Verification items for the finished model (mm, model axes). Face numbers are marked on the shaded views. A direction names the side the tool comes from. Give positions to 0.01 mm unless a question says otherwise; leave off trailing zeros. Order: outer loops, then holes, each group sorted by start corner. A loop starts at its lowest first (then second) coordinate and runs counter-clockwise, first axis right, second up. Notation, with made-up numbers: (20, 68.25) -> (78, 68.25) arc R9 ccw to (78, 78.25) -> close; hole circle Ø2 at (76, 17). An arc over 180 degrees is marked (long way). Return JSON: item names as keys, results as strings. Group by question number.
(1) Cross-section at C-C on y = 15. Enter the section's corners in (x, z), then the cut area to 3 significant figures.
(2) Cross-section at B-B on x = 1. Enter the section's corners in (y, z).
(3) Depth check by flat-ended pin: pin 1 Ø2.5 at (x, y) = (11, 19.05) entering from -Z; pin 2 Ø3 at (x, y) = (12.5, 19.5) entering from -Z; pin 3 Ø12 at (x, z) = (8.5, 5) entering from +Y; pin 4 Ø8 at (x, z) = (1, 24.5) entering from -Y. Enter the tip coordinate at first touch or a pass-through.
(4) Tool access check on the marked faces 1 and 2. Record the directions out of +Z, -Z, +X, -X, +Y, -Y that give a thin tool (end or side, any length) a straight path to the whole face; none if there is none.
(5) Cross-section at A-A on y = 0. Enter the section's corners in (x, z), then the cut area to 3 significant figures.
(6) Cross-section at D-D on x = -3.5. Enter the section's corners in (y, z), then the cut area to 3 significant figures.
(7) Thickness scan on line 1 along Y through (x, z) = (-11, 36); line 2 along Z through (x, y) = (0, -17.5); line 3 along X through (y, z) = (-10.5, 35). Record the ranges inside material, lowest first.
(8) Release check for a two-part mould opening along Y. For the marked faces 3, 4 and 5 record: pulls with the +Y half, pulls with the -Y half, needs draft (parallel to the pull), parting line crosses it, or undercut.
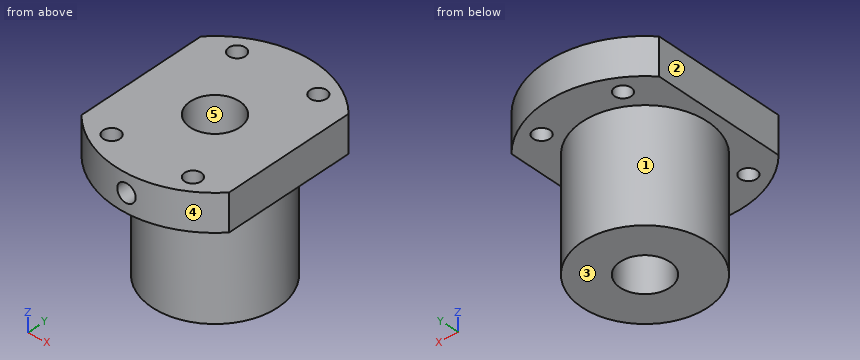
from build123d import *

# Parameters (mm, degrees)
SKETCH1_R                        = 17
BOSS_EXTRUDE1_DEPTH              = 30
BOSS_EXTRUDE2_DEPTH              = 10
SKETCH4_R                        = 6.71
CUT_EXTRUDE1_DEPTH               = 53.239831546
TAP_DRILL_FOR_M6X1_0_TAP1_REACH  = 72.114
TAP_DRILL_FOR_M6X1_0_TAP1_BORE_R = 2.5
F_4_5_4_5_DIAMETER_HOLE1_D       = 4.5


with BuildPart() as part:
    # Sketch1 → Boss-Extrude1 (new body)
    with BuildSketch(Plane.XY):
        Circle(SKETCH1_R)
    extrude(amount=BOSS_EXTRUDE1_DEPTH)

    # Sketch3 → Boss-Extrude2 (add)
    with BuildSketch(Plane.XY.offset(30)):
        with BuildLine():
            Line((-20, -18.138357147), (-20, 18.138357147))
            ThreePointArc((-20, 18.138357147), (0, 27), (20, 18.138357147))
            Line((20, 18.138357147), (20, -18.138357147))
            ThreePointArc((20, -18.138357147), (0, -27), (-20, -18.138357147))
        make_face()
    extrude(amount=BOSS_EXTRUDE2_DEPTH)

    # Sketch4 → Cut-Extrude1 (cut, through all)
    with BuildSketch(Plane.XY.offset(40)):
        Circle(SKETCH4_R)
    extrude(amount=-CUT_EXTRUDE1_DEPTH, mode=Mode.SUBTRACT)

    # Tap Drill for M6x1.0 Tap1 bore → Tap Drill for M6x1.0 Tap1 (cut, up to next)
    with BuildSketch(Plane(origin=(0, -27, 0), x_dir=(-1, 0, 0), z_dir=(0, -1, 0)), mode=Mode.PRIVATE) as tap_drill_for_m6x1_0_tap1_sk1:
        with Locations((0, -35)):
            Circle(TAP_DRILL_FOR_M6X1_0_TAP1_BORE_R)
    tap_drill_for_m6x1_0_tap1_tool1 = extrude(tap_drill_for_m6x1_0_tap1_sk1.sketch, amount=-TAP_DRILL_FOR_M6X1_0_TAP1_REACH, mode=Mode.PRIVATE) & part.part
    add(tap_drill_for_m6x1_0_tap1_tool1.solids().sort_by_distance((0, -27, 35))[0], mode=Mode.SUBTRACT)

    # Ø4.5 (4.5) Diameter Hole1 (through all)
    with Locations(Plane.XY.offset(40)):
        with Locations((-11, -19.052558883), (-11, 19.052558883), (11, 19.052558883), (11, -19.052558883)):
            Hole(F_4_5_4_5_DIAMETER_HOLE1_D / 2)


solid = part.part
Verdict:
{
 "1": {"outline": "(-20, 30) -> (-8, 30) -> (-8, 0) -> (8, 0) -> (8, 30) -> (20, 30) -> (20, 40) -> (-20, 40) -> close", "area": "880 mm²"},
 "2": {"outline": "(-26.98, 30) -> (-16.97, 30) -> (-16.97, 0) -> (-6.64, 0) -> (-6.64, 32.71) -> (-26.98, 32.71) -> close; (-26.98, 37.29) -> (-6.64, 37.29) -> (-6.64, 40) -> (-26.98, 40) -> close; (6.64, 0) -> (16.97, 0) -> (16.97, 30) -> (26.98, 30) -> (26.98, 40) -> (6.64, 40) -> close"},
 "3": {"pin 1": "through", "pin 2": "z = 30", "pin 3": "y = 16.82", "pin 4": "y = -17"},
 "4": {"face 1": "-Z", "face 2": "+Z, -Z, -X, +Y, -Y"},
 "5": {"outline": "(-20, 30) -> (-17, 30) -> (-17, 0) -> (-6.71, 0) -> (-6.71, 40) -> (-20, 40) -> close; (6.71, 0) -> (17, 0) -> (17, 30) -> (20, 30) -> (20, 40) -> (6.71, 40) -> close", "area": "883 mm²"},
 "6": {"outline": "(-26.77, 30) -> (-16.64, 30) -> (-16.64, 0) -> (-5.72, 0) -> (-5.72, 40) -> (-26.77, 40) -> close; (5.72, 0) -> (16.64, 0) -> (16.64, 30) -> (26.77, 30) -> (26.77, 40) -> (5.72, 40) -> close", "area": "1,080 mm²"},
 "7": {"line 1": "-24.66 to -21.3, -16.8 to 16.8, 21.3 to 24.66", "line 2": "30 to 32.5, 37.5 to 40", "line 3": "-20 to -2.5, 2.5 to 20"},
 "8": {"face 3": "needs draft", "face 4": "pulls with the -Y half", "face 5": "undercut"}
}
